Model file for the job. Use its own axes, mm. A direction names the side the tool comes from. Coordinates: 2 decimals unless noted, no trailing zeros. Write each loop counter-clockwise with the first axis right and the second up, starting at its lowest first coordinate (ties: lowest second). Pieces come first, ordered by that corner, then holes. Notation, with made-up numbers: (69.25, -1.75) - (90.25, -1.75) arc R21 ccw to (90.25, 28.25) - close; hole circle Ø9 at (25.5, 11). An arc over 180 degrees is marked (long way). Put each result on its own line as item: value. Start each with the question number.
1. Saw through at A-A, the plane z = 11. Write the cut outline in (x, y).
2. Pull direction X, two halves, no side cores. Call faces 4 (the face through (-3, 2, 18)), 5 (the face through (13.199, 7.215, 29.754)), 6 (the face through (20, 1, 17)): released by +X, released by -X, zero draft, split by the parting line, or undercut.
3. Drop flat-ended pins along their axis: P1, Ø5, axis at y = 6, z = 16.5, coming from the +X side; P2, Ø7, axis at y = 6, z = 21, coming from the +X side; P3, Ø2.5, axis at y = 3.5, z = 18, coming from the +X side. Give the stop position or say it passes through.
4. Saw through at C-C, the plane x = 17.5. Write the cut outline in (y, z), plus the area to 3 significant figures.
5. Which spindle directions (+Z, -Z, +X, -X, +Y, -Y) get a long thin tool onto all of the face, cutting with end or side? Do faces 1 (the face through (0, 7, 17)), 2 (the face through (1.785, 9.699, 17.332)), 3 (the face through (1.785, 7.199, 5.254)). Say none if no direction does.
6. Saw through at D-D, the plane y = 8.25. Write the cut outline in (x, z).
7. Saw through at B-B, the plane y = 5.5. Write the cut outline in (x, z), plus the area to 3 significant figures.
8. Drill centre lines: L1, parallel to X at y = 0.7, z = 11; L2, parallel to X at y = 1, z = 14.25; L3, parallel to X at y = 8.5, z = 29. Where is each one in solid material? Low to high. Write a range as from..to.
```python
from build123d import *

# Parameters (mm, degrees)
SKETCH1_W               = 15
SKETCH1_H               = 12
BOSS_EXTRUDE1_DEPTH     = 30
SKETCH3_W               = 12
SKETCH3_H               = 10
CUT_EXTRUDE1_DEPTH      = 30
FILLET1_R               = 1
SKETCH4_W               = 12
SKETCH4_H               = 0.5
BOSS_EXTRUDE3_DEPTH     = 2.5
CUT_EXTRUDE2_DEPTH      = 36.623026261
CUT_EXTRUDE2_DEPTH_BACK = 36.623026261
SKETCH5_W               = 15
SKETCH5_H               = 5
SKETCH6_W               = 5
SKETCH6_H               = 25
SKETCH6_R               = 1.162975042
SKETCH6_R_2             = 1.164851314
BOSS_EXTRUDE4_DEPTH     = 2
FILLET2_R               = 1


with BuildPart() as part:
    # Sketch1 → Boss-Extrude1 (new body)
    with BuildSketch(Plane.XY):
        with Locations((7.5, 6)):
            Rectangle(SKETCH1_W, SKETCH1_H)
    extrude(amount=BOSS_EXTRUDE1_DEPTH)

    # Sketch3 → Cut-Extrude1 (cut)
    with BuildSketch(Plane.XY.offset(30)):
        with Locations((7.5, 5)):
            Rectangle(SKETCH3_W, SKETCH3_H)
    extrude(amount=-CUT_EXTRUDE1_DEPTH, mode=Mode.SUBTRACT)

    # Fillet1
    fillet1_edges = [part.edges().sort_by_distance(p)[0] for p in [
        (1.5, 10, 15),
        (13.5, 10, 15),
    ]]
    fillet(fillet1_edges, radius=FILLET1_R)

    # Sketch4 → Boss-Extrude3 (add)
    with BuildSketch(Plane.XZ.offset(-10)):
        with Locations((7.5, 29.75)):
            Rectangle(SKETCH4_W, SKETCH4_H)
        with Locations((7.5, 5.25)):
            Rectangle(SKETCH4_W, SKETCH4_H)
    extrude(amount=BOSS_EXTRUDE3_DEPTH)

    # Sketch5 → Cut-Extrude2 (cut, two sides: drawn at the far end of the back side and taken through both)
    with BuildSketch(Plane.XZ.offset(-CUT_EXTRUDE2_DEPTH_BACK)):
        with Locations((7.5, 2.5)):
            Rectangle(SKETCH5_W, SKETCH5_H)
    extrude(amount=CUT_EXTRUDE2_DEPTH + CUT_EXTRUDE2_DEPTH_BACK, mode=Mode.SUBTRACT)

    # Sketch6 → Boss-Extrude4 (add)
    # profile 1 of 2: a face of its own
    with BuildSketch(Plane.XZ):
        with Locations((17.5, 17.5)):
            Rectangle(SKETCH6_W, SKETCH6_H)
        with Locations(Location((17.5, 24, 0), (0, 0, 270))):
            Circle(SKETCH6_R, mode=Mode.SUBTRACT)
        with Locations(Location((17.5, 11, 0), (0, 0, 270))):
            Circle(SKETCH6_R_2, mode=Mode.SUBTRACT)
    # profile 2 of 2: a face of its own
    with BuildSketch(Plane.XZ):
        with Locations((-2.5, 17.5)):
            Rectangle(SKETCH6_W, SKETCH6_H)
        with Locations(Location((-2.5, 11, 0), (0, 0, 90))):
            Circle(SKETCH6_R_2, mode=Mode.SUBTRACT)
        with Locations(Location((-2.5, 24, 0), (0, 0, 90))):
            Circle(SKETCH6_R, mode=Mode.SUBTRACT)
    extrude(amount=-BOSS_EXTRUDE4_DEPTH)

    # Fillet2
    fillet2_edges = [part.edges().sort_by_distance(p)[0] for p in [
        (15, 2, 17.5),
        (20, 1, 30),
        (20, 1, 5),
        (0, 2, 17.5),
        (-5, 1, 5),
        (-5, 1, 30),
        (13.5, 7.5, 29.75),
        (1.5, 7.5, 29.75),
        (13.5, 7.5, 5.25),
        (1.5, 7.5, 5.25),
    ]]
    fillet(fillet2_edges, radius=FILLET2_R)


solid = part.part
```
Final values:
1. outline: (-5, 0) - (-3.66, 0) - (-3.66, 2) - (-5, 2) - close; (-1.34, 0) - (1.5, 0) - (1.5, 9) arc R1 cw to (2.5, 10) - (12.5, 10) arc R1 cw to (13.5, 9) - (13.5, 0) - (16.34, 0) - (16.34, 2) - (16, 2) arc R1 cw to (15, 3) - (15, 12) - (0, 12) - (0, 3) arc R1 cw to (-1, 2) - (-1.34, 2) - close; (18.66, 0) - (20, 0) - (20, 2) - (18.66, 2) - close
2. face 4: zero draft
2. face 5: undercut
2. face 6: released by +X
3. P1: stops at x = 15
3. P2: stops at x = 15.13
3. P3: stops at x = 15.34
4. outline: (0, 5) - (2, 5) - (2, 9.84) - (0, 9.84) - close; (0, 12.16) - (2, 12.16) - (2, 22.84) - (0, 22.84) - close; (0, 25.16) - (2, 25.16) - (2, 30) - (0, 30) - close
4. area: 40.7 mm²
5. face 1: +Z, -Z, -X, +Y
5. face 2: -Y
5. face 3: +Z, -Z, -Y
6. outline: (0, 5) - (15, 5) - (15, 30) - (0, 30) - close; hole (1.5, 5.5) - (13.5, 5.5) - (13.5, 29.5) - (1.5, 29.5) - close
7. outline: (0, 5) - (1.5, 5) - (1.5, 30) - (0, 30) - close; (13.5, 5) - (15, 5) - (15, 30) - (13.5, 30) - close
7. area: 75.0 mm²
8. L1: x = -5..-3.66, -1.34..1.5, 13.5..16.34, 18.66..20
8. L2: x = -5..1.5, 13.5..20
8. L3: x = 0..1.5, 13.5..15
